Source: CAD feature listing. Evaluate the final solid. Frame: model axes, mm. A direction names the side the tool comes from. Round coordinates to 2 decimals unless told otherwise and drop trailing zeros. Order: outer loops, then holes, each group sorted by start corner. A loop starts at its lowest first (then second) coordinate and runs counter-clockwise, first axis right, second up. Notation, with made-up numbers: (-39.75, 17) - (-10.75, 17) arc R19 ccw to (-10.75, 40) - close; hole circle Ø2 at (-4, -14). An arc over 180 degrees is marked (long way). Put each result on its own line as item: value. Start each with the question number.
1) Section A-A on z = 5. Output: boundary loops of the cut face in (x, y).
2) Mould query, pull axis X, two halves, no side actions, for faces 1 (the face through (-42, -28, 0)), 2 (the face through (-40.046, -26.674, 1.726)), 3 (the face through (-43.877, -24.474, 11.358)), 4 (the face through (-41.98, -22.228, 1.038)). Classes: +X half, -X half, draft (parallel to the pull), parting line (faces both ways), or undercut.
3) Section B-B on z = 10.5. Output: boundary loops of the cut face in (x, y).
4) Contact query for flat-ended pins moving along their axis: P1, Ø5, axis at y = -22.5, z = 2, coming from the -X side; P2, Ø3, axis at x = -41.5, y = -26.07, coming from the +Z side; P3, Ø4, axis at x = -44, z = 4.5, coming from the -Y side; P4, Ø3, axis at y = -21, z = 8.5, coming from the +X side. Output: stop coordinate, or through.
5) Line query: probe 1 along Y at (x, z) = (-42.5, 4.25); probe 2 along Z at (x, y) = (-40.25, -28.25); probe 3 along X at (y, z) = (-24.5, 7). Output: solid intervals per line, ascending. Write a range as [from, to].
6) Access query for faces 5 (the face through (-46, -25, 14)), 6 (the face through (-41.04, -32.75, 16.29)), 7 (the face through (-40, -27, 3.5)). Directions: +Z, -Z, +X, -X, +Y, -Y. A direction counts if a zero-diameter tool reaches every point of the face in a straight line with its end or side. Return the directions, or none.
```python
from build123d import *

# Parameters (mm, degrees)
F0_R         = 3.9
F2_DEPTH     = 14
F3_R         = 7.5
F4_DEPTH     = 5
F6_R         = 4.3
F7_DEPTH     = 4.1
F1_R         = 1.5693660879
F8_DEPTH     = 23.4
F9_DEPTH     = 15.5
F10_R        = 0.2
F11_S5_R     = 4.3
F11_T6_DEPTH = 9
F12_R        = 1.5
F13_R        = 2.5
F15_R        = 8.6051956913
F16_DEPTH    = 6


# Not quite as in the source:
# - a fillet or chamfer that OpenCascade refuses, or shapes differently, is made with other operations: its cross-section is extruded or revolved along the edge and cut away or added


with BuildPart() as f2:
    # F0 (on Top) → F2 (new body)
    with BuildSketch(Plane.XY):
        with Locations((-41.4718948305, -26.0946750641)):
            Circle(F0_R)
    extrude(amount=F2_DEPTH)

    # F3 (on face) → F4 (join)
    with BuildSketch(Plane.XY.offset(14)):
        with Locations((-41.4718948305, -26.0946750641)):
            Circle(F3_R)
    extrude(amount=F4_DEPTH)

    # F6 (on face) → F7 (join)
    with BuildSketch(Plane(origin=(0, 0, 14), x_dir=(1, 0, 0), z_dir=(0, 0, -1))):
        with Locations((-41.4718948305, 26.0946750641)):
            Circle(F6_R)
    extrude(amount=F7_DEPTH)

    # F1 (on Top) → F8 (cut)
    with BuildSketch(Plane.XY):
        with Locations((-41.495975107, -26.0728988796)):
            Circle(F1_R)
    extrude(amount=F8_DEPTH, mode=Mode.SUBTRACT)

    # F5 (on face) → F9 (cut)
    with BuildSketch(Plane.XY.offset(19)):
        Polygon((-39.9783341683, -29.0917753096), (-38.1295495491, -26.2997637113), (-39.6231102113, -23.3026634658), (-42.9654554927, -23.0975748186), (-44.8142401119, -25.8895864169), (-43.3206794497, -28.8866866624), align=None)
    extrude(amount=-F9_DEPTH, mode=Mode.SUBTRACT)

    # F10
    f10_edges = [f2.edges().sort_by_distance(p)[0] for p in [
        (-45.371895, -26.094675, 0),
    ]]
    fillet(f10_edges, radius=F10_R)

    # F11: chamfer of 8 x 0.4612770977 on 1 edges, made by hand


with BuildPart() as f11_tool2:
    # F11_s3 → F11_t4 (revolve)
    with BuildSketch(Plane.XZ.offset(26.0946750641)):
        Polygon((-37.5718948305, 1.9), (-37.1106177328, 9.9), (-37.5718948305, 9.9), align=None)
    revolve(axis=Axis((-41.4718948305, -26.0946750641, 9.9), (0, 0, -1)))

    # F11_s5 → F11_t6 (intersect, symmetric)
    with BuildSketch(Plane.XY.offset(5.9)):
        with Locations((-41.4718948305, -26.0946750641)):
            Circle(F11_S5_R)
    extrude(amount=F11_T6_DEPTH, both=True, mode=Mode.INTERSECT)


with BuildPart() as f2_1:
    add(f2.part)

    # F11_t1: union F11_tool2
    add(f11_tool2.part)

    # F12
    f12_edges = [f2_1.edges().sort_by_distance(p)[0] for p in [
        (-48.971895, -26.094675, 14),
    ]]
    fillet(f12_edges, radius=F12_R)

    # F13
    f13_edges = [f2_1.edges().sort_by_distance(p)[0] for p in [
        (-48.971895, -26.094675, 19),
    ]]
    fillet(f13_edges, radius=F13_R)

    # F15 (on face) → F16 (cut)
    with BuildSketch(Plane.XY.offset(19)):
        with Locations((-41.4718948305, -26.0946750641)):
            Circle(F15_R)
        Polygon((-49.1588137584, -26.5433145587), (-45.7038874939, -19.661927743), (-38.016968566, -19.2132882484), (-33.7849759026, -25.6460355695), (-37.2399021671, -32.5274223852), (-44.926821095, -32.9760618798), align=None, mode=Mode.SUBTRACT)
    extrude(amount=-F16_DEPTH, mode=Mode.SUBTRACT)


solid = f2_1.part
```
Answer sheet:
1. outline: circle Ø8.16 at (-41.47, -26.09); hole (-44.81, -25.89) - (-43.32, -28.89) - (-39.98, -29.09) - (-38.13, -26.3) - (-39.62, -23.3) - (-42.97, -23.1) - close
2. face 1: draft
2. face 2: undercut
2. face 3: undercut
2. face 4: parting line
3. outline: circle Ø8.6 at (-41.47, -26.09); hole (-44.81, -25.89) - (-43.32, -28.89) - (-39.98, -29.09) - (-38.13, -26.3) - (-39.62, -23.3) - (-42.97, -23.1) - close
4. P1: x = -45.24
4. P2: through
4. P3: y = -30.13
4. P4: x = -39.14
5. probe 1: [-30, -28.94], [-23.13, -22.19]
5. probe 2: [0, 3.5]
5. probe 3: [-45.35, -43.89], [-39.03, -37.59]
6. face 5: -Z
6. face 6: +Z, -Z, +X, -Y
6. face 7: +Z
